The listing builds one solid part. Answer for the finished solid, in the listing's coordinates (mm). A direction names the side the tool comes from. Coordinates: 2 decimals unless noted, no trailing zeros. Loops run counter-clockwise (first coordinate to the right, second up) from the corner with the lowest first, then second, coordinate; pieces in that order, holes last. Notation, with made-up numbers: (-1.75, 12) - (57.25, 12) arc R10 cw to (57.25, 28) - close; hole circle Ø10 at (80, 86.25). An arc over 180 degrees is marked (long way). Return JSON: item names as keys, results as strings. Group by question number.
1. This flat-tipped pin is pushed along its axis until it touches: P1, Ø10, axis at x = 49, y = 20.5, coming from the -Z side. Where does it stop, or does it pass through?
2. Section D-D (y = 25.25) is taken. Write down the section's boundary in (x, z), and give its area (3 significant figures).
3. Section A-A (x = 67) is taken. Write down the section's boundary in (y, z).
4. Section B-B (z = 4.25) is taken. Write down the section's boundary in (x, y).
5. Which of the six approach directions +Z, -Z, +X, -X, +Y, -Y give full straight-line access (tool end or side, diameter ignored) to faces 5 (the face through (50, 11, 13)), 6 (the face through (49, 20, 11)), 7 (the face through (34.751, 20, 2))?
6. Find the intervals of material crossed by line 1 along Y through (x, z) = (41.5, 12.5); line 2 along X through (y, z) = (24.25, 4.5); line 3 along Z through (x, y) = (72, 25.25), in increasing order.
7. The mould has two halves that part along Y. Classify faces 1 (the face through (75.503, 20, 7)), 2 (the face through (49, 31.8, 8)), 3 (the face through (50, 8.2, 8)), 4 (the face through (50, 14, 12)): pulls with the +Y half, pulls with the -Y half, needs draft (parallel to the pull), parting line crosses it, or undercut.
8. Section C-C (y = 29.25) is taken. Write down the section's boundary in (x, z), and give its area (3 significant figures).
```python
from build123d import *

# Parameters (mm, degrees)
CROQUIS2_W              = 51.502836605
CROQUIS2_H              = 23.6
SALIENTE_EXTRUIR1_DEPTH = 11
CROQUIS4_W              = 2
CROQUIS4_H              = 5.8
SALIENTE_EXTRUIR2_DEPTH = 51.502837
CORTAR_EXTRUIR1_START   = -23.6
CORTAR_EXTRUIR1_DEPTH   = 23.6


with BuildPart() as part:
    # Croquis2 → Saliente-Extruir1 (new body)
    with BuildSketch(Plane.XY):
        with Locations((49.751418302, 20)):
            Rectangle(CROQUIS2_W, CROQUIS2_H)
    extrude(amount=SALIENTE_EXTRUIR1_DEPTH)

    # Croquis4 → Saliente-Extruir2 (add)
    with BuildSketch(Plane(origin=(75.502836605, 0, 0), x_dir=(0, 0, -1), z_dir=(1, 0, 0))):
        with Locations((-12, 11.1)):
            Rectangle(CROQUIS4_W, CROQUIS4_H)
        with Locations((-12, 28.9)):
            Rectangle(CROQUIS4_W, CROQUIS4_H)
    extrude(amount=-SALIENTE_EXTRUIR2_DEPTH)

    # Croquis5 → Cortar-Extruir1 (cut)
    with BuildSketch(Plane.XZ.offset(-8.2).offset(CORTAR_EXTRUIR1_START)):
        Polygon((49.751418302, 0), (34.751418302, 0), (34.751418302, 5), (49.751418302, 5), (64.751418302, 5), (64.751418302, 0), align=None)
    extrude(amount=CORTAR_EXTRUIR1_DEPTH, mode=Mode.SUBTRACT)


solid = part.part
```
The answers:
{
 "1": {"P1": "stops at z = 5"},
 "2": {"outline": "(24, 0) - (34.75, 0) - (34.75, 5) - (64.75, 5) - (64.75, 0) - (75.5, 0) - (75.5, 11) - (24, 11) - close", "area": "417 mm2"},
 "3": {"outline": "(8.2, 0) - (31.8, 0) - (31.8, 13) - (26, 13) - (26, 11) - (14, 11) - (14, 13) - (8.2, 13) - close"},
 "4": {"outline": "(24, 8.2) - (34.75, 8.2) - (34.75, 31.8) - (24, 31.8) - close; (64.75, 8.2) - (75.5, 8.2) - (75.5, 31.8) - (64.75, 31.8) - close"},
 "5": {"face 5": "+Z, +X, -X, +Y, -Y", "face 6": "+Z, +X, -X", "face 7": "-Z, +Y, -Y"},
 "6": {"line 1": "y = 8.2 to 14, 26 to 31.8", "line 2": "x = 24 to 34.75, 64.75 to 75.5", "line 3": "z = 0 to 11"},
 "7": {"face 1": "needs draft", "face 2": "pulls with the +Y half", "face 3": "pulls with the -Y half", "face 4": "undercut"},
 "8": {"outline": "(24, 0) - (34.75, 0) - (34.75, 5) - (64.75, 5) - (64.75, 0) - (75.5, 0) - (75.5, 13) - (24, 13) - close", "area": "520 mm2"}
}
